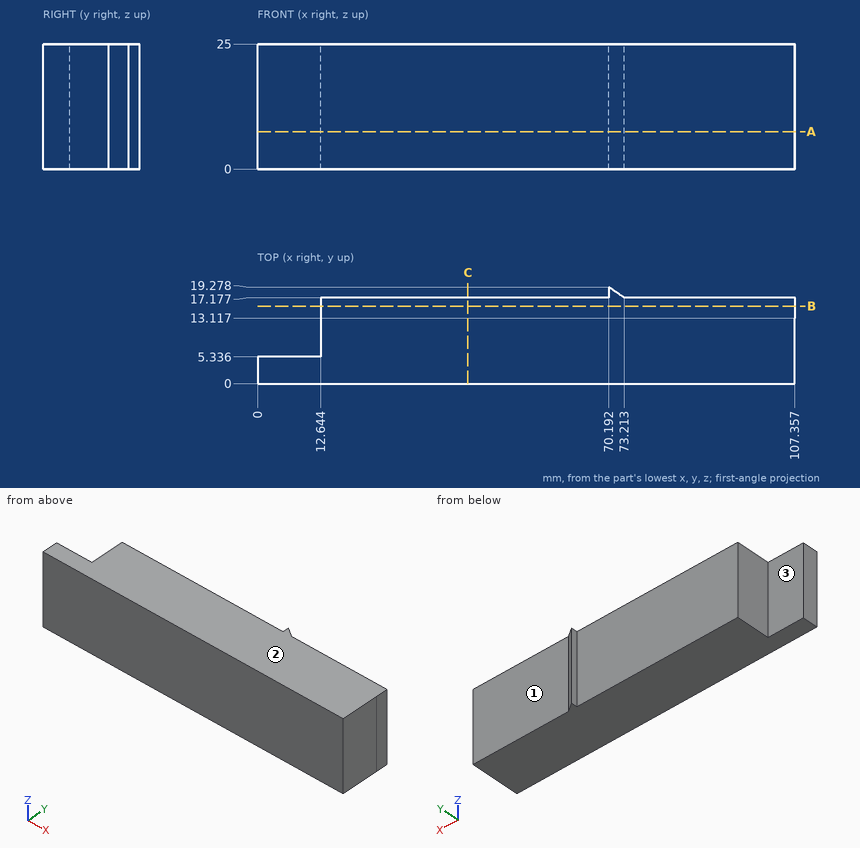
For this review, use the dimensioned drawing (mm, ordinates from the lowest corner) and the shaded views. A direction names the side the tool comes from. Coordinates: 2 decimals unless noted, no trailing zeros. Loops run counter-clockwise (first coordinate to the right, second up) from the corner with the lowest first, then second, coordinate; pieces in that order, holes last.
1. For the marked faces 1, 2 and 3, list the 3-axis set-ups (+Z, -Z, +X, -X, +Y, -Y) from which the entire face can be reached by the end or side of a thin tool; tool diameter is ignored.
2. Insertion check: P1, Ø12.5, axis at x = 82, z = 16, coming from the +Y side; P2, Ø2, axis at x = 62.5, y = 10, coming from the -Z side; P3, Ø1, axis at y = 12, z = 13.5, coming from the -X side; P4, Ø0.6, axis at y = 18.5, z = 8.5, coming from the -X side. Each pin has a flat end and moves straight along its axis. Give the tip position at first contact, or say it passes through.
3. Add section C-C, the plane x = 42. Give the boundary of the cut face in (y, z).
4. Add section B-B, the plane y = 15.5. Give the boundary of the cut face in (x, z) (1 decimal).
5. Add section A-A, the plane z = 7.5. Give the boundary of the cut face in (x, y) (1 decimal).
6. For line 1 (Y direction, x = 13.5, z = 4.5); line 2 (X direction, y = 8.5, z = 21.5) (1 decimal), list the stretches that pass through material, from the lowest coordinate up.
Result:
1. face 1: +Z, -Z, +X, +Y
1. face 2: +Z, +X, -X, +Y, -Y
1. face 3: +Z, -Z, -X, +Y
2. P1: stops at y = 17.18
2. P2: stops at z = 0
2. P3: stops at x = 12.64
2. P4: stops at x = 70.19
3. outline: (0, 0) - (17.18, 0) - (17.18, 25) - (0, 25) - close
4. outline: (12.6, 0) - (107.4, 0) - (107.4, 25) - (12.6, 25) - close
5. outline: (0, 0) - (107.4, 0) - (107.4, 17.2) - (73.2, 17.2) - (70.2, 19.3) - (70.2, 17.2) - (12.6, 17.2) - (12.6, 5.3) - (0, 5.3) - close
6. line 1: y = 0 to 17.18
6. line 2: x = 12.6 to 107.4
